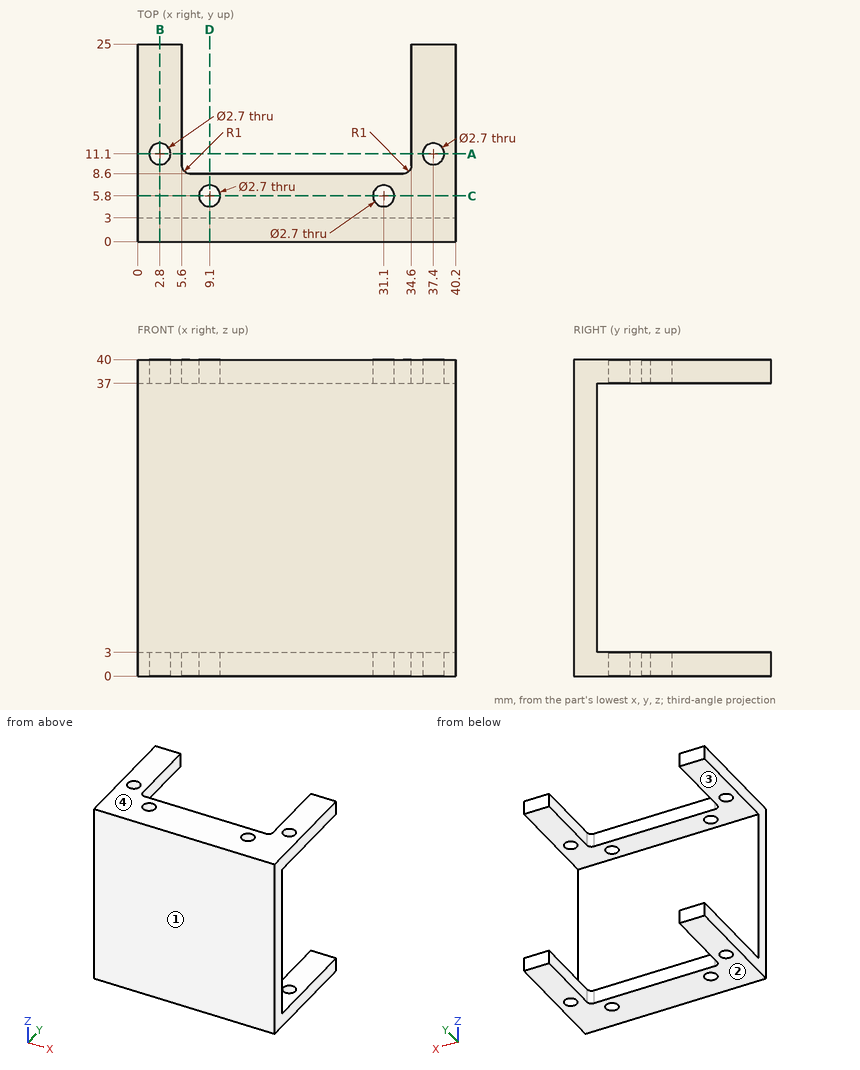
Drawing for the job (mm, zero at the part's lowest x, y, z). Give positions to 0.01 mm unless a question says otherwise; leave off trailing zeros. Order: outer loops, then holes, each group sorted by start corner. A loop starts at its lowest first (then second) coordinate and runs counter-clockwise, first axis right, second up. Notation, with made-up numbers: (29.5, -3.5) - (88.5, -3.5) arc R21 ccw to (88.5, 3.5) - close; hole circle Ø7 at (81, 61). An arc over 180 degrees is marked (long way). Write item = value, one per line. Start each with the question number.
1. Cut at C-C, the plane y = 5.8. List the corners of the cut face in (x, z).
2. Drop flat-ended pins along their axis: P1, Ø2.5, axis at x = 31.1, y = 5.8, coming from the +Z side; P2, Ø2.5, axis at x = 26, z = 1, coming from the +Y side. Give the stop position or say it passes through.
3. Cut at D-D, the plane x = 9.1. List the corners of the cut face in (y, z).
4. Cut at A-A, the plane y = 11.1. State how many separate pieces and enclosed holes the cut face has, and give its area (3 significant figures).
5. Probe line 1 along X through (y, z) = (11.1, 38.65); line 2 along X through (y, z) = (5.8, 0.9); line 3 along Y through (x, z) = (37.4, 39.1). List the from-to ranges inside material, lowest first.
6. Two-plate mould, pull along Z, no slides. Class the marked faces 1, 2, 3 and 4: pulls with the +Z half, pulls with the -Z half, needs draft (parallel to the pull), parting line crosses it, or undercut.
7. Cut at B-B, the plane x = 2.8. List the corners of the cut face in (y, z).
Taken from the geometry:
q1.outline = (0, 0) - (7.75, 0) - (7.75, 3) - (0, 3) - close; (0, 37) - (7.75, 37) - (7.75, 40) - (0, 40) - close; (10.45, 0) - (29.75, 0) - (29.75, 3) - (10.45, 3) - close; (10.45, 37) - (29.75, 37) - (29.75, 40) - (10.45, 40) - close; (32.45, 0) - (40.2, 0) - (40.2, 3) - (32.45, 3) - close; (32.45, 37) - (40.2, 37) - (40.2, 40) - (32.45, 40) - close
q2.P1 = through
q2.P2 = 8.6
q3.outline = (0, 0) - (4.45, 0) - (4.45, 3) - (3, 3) - (3, 37) - (4.45, 37) - (4.45, 40) - (0, 40) - close; (7.15, 0) - (8.6, 0) - (8.6, 3) - (7.15, 3) - close; (7.15, 37) - (8.6, 37) - (8.6, 40) - (7.15, 40) - close
q4.separate_pieces = 8
q4.enclosed_holes = 0
q4.area = 34.8 mm²
q5.line_1 = 0 to 1.45, 4.15 to 5.6, 34.6 to 36.05, 38.75 to 40.2
q5.line_2 = 0 to 7.75, 10.45 to 29.75, 32.45 to 40.2
q5.line_3 = 0 to 9.75, 12.45 to 25
q6.face_1 = needs draft
q6.face_2 = pulls with the -Z half
q6.face_3 = undercut
q6.face_4 = pulls with the +Z half
q7.outline = (0, 0) - (9.75, 0) - (9.75, 3) - (3, 3) - (3, 37) - (9.75, 37) - (9.75, 40) - (0, 40) - close; (12.45, 0) - (25, 0) - (25, 3) - (12.45, 3) - close; (12.45, 37) - (25, 37) - (25, 40) - (12.45, 40) - close
